Read the model definition and answer for the solid it produces. Units are mm, in the model's axes. Face numbers are marked on the shaded views. A direction names the side the tool comes from. Round coordinates to 2 decimals unless told otherwise and drop trailing zeros. Order: outer loops, then holes, each group sorted by start corner. A loop starts at its lowest first (then second) coordinate and runs counter-clockwise, first axis right, second up.
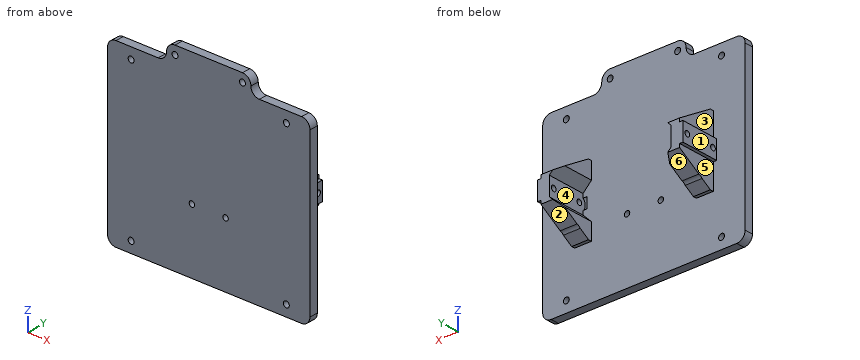
from build123d import *

# Parameters (mm, degrees)
EXTRUDE_1_DEPTH         = 5
FILLET_1_R              = 5
SKETCH_2_W              = 7
SKETCH_2_H              = 11
EXTRUDE_2_DEPTH         = 23
SKETCH_3_R              = 1.6
CUT_EXTRUDE_1_DEPTH     = 119.006186279
SKETCH_5_R              = 1.75
CUT_EXTRUDE_3_DEPTH     = 90.639556001
SKETCH_6_R              = 1.75
CUT_EXTRUDE_4_DEPTH     = 90.639556001
SKETCH2_R               = 4
CUT_EXTRUDE1_DEPTH      = 2.5
CUT_EXTRUDE2_START      = 2.5
SKETCH3_R               = 4
CUT_EXTRUDE2_DEPTH      = 2.5
CUT_EXTRUDE3_DEPTH      = 90.639556001
CUT_EXTRUDE3_DEPTH_BACK = 90.639556001
SKETCH4_R               = 1.6
EXTRUDE_4_DEPTH         = 5
EXTRUDE_4_DEPTH_BACK    = 5
EXTRUDE_5_DEPTH         = 5
EXTRUDE_5_DEPTH_BACK    = 5
CHAMFER_1_SIZE          = 5
SKETCH_12_R             = 1.6
EXTRUDE_6_DEPTH         = 5


with BuildPart() as part:
    # Sketch 1 → Extrude 1 (new body)
    with BuildSketch(Plane(origin=(0, 0, 0), x_dir=(1, 0, 0), z_dir=(0, 1, 0))):
        Polygon((-25, -52.5), (-60, -52.5), (-60, 52.5), (60, 52.5), (60, -52.5), (25, -52.5), (25, -62.5), (-25, -62.5), align=None)
    extrude(amount=EXTRUDE_1_DEPTH)

    # Fillet 1
    fillet_1_edges = [part.edges().sort_by_distance(p)[0] for p in [
        (60, 2.5, -52.5),
        (60, 2.5, 52.5),
        (-60, 2.5, -52.5),
        (-60, 2.5, 52.5),
        (-25, 2.5, 52.5),
        (25, 2.5, 52.5),
        (25, 2.5, 62.5),
        (-25, 2.5, 62.5),
    ]]
    fillet(fillet_1_edges, radius=FILLET_1_R - 0.0001)  # a hair under: the kernel refuses the full size

    # Sketch 5 → Cut-Extrude 3 (cut, through all)
    with BuildSketch(Plane(origin=(0, 5, 0), x_dir=(1, 0, 0), z_dir=(0, 1, 0))):
        with Locations(Location((-46, -46, 0), (0, 0, 270))):
            Circle(SKETCH_5_R)
        with Locations(Location((-46, 46, 0), (0, 0, 270))):
            Circle(SKETCH_5_R)
        with Locations(Location((46, 46, 0), (0, 0, 270))):
            Circle(SKETCH_5_R)
        with Locations(Location((46, -46, 0), (0, 0, 270))):
            Circle(SKETCH_5_R)
    extrude(amount=-CUT_EXTRUDE_3_DEPTH, mode=Mode.SUBTRACT)

    # Sketch 6 → Cut-Extrude 4 (cut, through all)
    with BuildSketch(Plane(origin=(0, 5, 0), x_dir=(1, 0, 0), z_dir=(0, 1, 0))):
        with Locations(Location((20, -57.5, 0), (0, 0, 270))):
            Circle(SKETCH_6_R)
        with Locations(Location((-20, -57.5, 0), (0, 0, 270))):
            Circle(SKETCH_6_R)
    extrude(amount=-CUT_EXTRUDE_4_DEPTH, mode=Mode.SUBTRACT)

    # Sketch2 → Cut-Extrude1 (cut)
    with BuildSketch(Plane.ZY.offset(-36.1)):
        with Locations((-0.7, 7.5)):
            Circle(SKETCH2_R)
    extrude(amount=CUT_EXTRUDE1_DEPTH, mode=Mode.SUBTRACT)

    # Sketch3 → Cut-Extrude2 (cut)
    with BuildSketch(Plane(origin=(-36.1, 0, 0), x_dir=(0, 0, -1), z_dir=(1, 0, 0)).offset(CUT_EXTRUDE2_START)):
        with Locations((0.7, 7.5)):
            Circle(SKETCH3_R)
    extrude(amount=-CUT_EXTRUDE2_DEPTH, mode=Mode.SUBTRACT)

    # Sketch4 → Cut-Extrude3 (cut, two sides: drawn at the far end of the back side and taken through both)
    with BuildSketch(Plane(origin=(0, 5, 0), x_dir=(1, 0, 0), z_dir=(0, 1, 0)).offset(-CUT_EXTRUDE3_DEPTH_BACK)):
        with Locations(Location((-10, 0, 0), (0, 0, 270))):
            Circle(SKETCH4_R)
        with Locations(Location((10, 0, 0), (0, 0, 270))):
            Circle(SKETCH4_R)
        with Locations(Location((-10, 14.7, 0), (0, 0, 270))):
            Circle(SKETCH4_R)
        with Locations(Location((10, 14.7, 0), (0, 0, 270))):
            Circle(SKETCH4_R)
    extrude(amount=CUT_EXTRUDE3_DEPTH + CUT_EXTRUDE3_DEPTH_BACK, mode=Mode.SUBTRACT)



with BuildPart() as body_2:
    # Sketch 2 → Extrude 2 (new body)
    with BuildSketch(Plane(origin=(0, 5, 0), x_dir=(1, 0, 0), z_dir=(0, 1, 0))):
        with Locations((-39.6, 0.7)):
            Rectangle(SKETCH_2_W, SKETCH_2_H)
    extrude(amount=EXTRUDE_2_DEPTH)

    # Sketch 3 → Cut-Extrude 1 (cut, through all)
    with BuildSketch(Plane(origin=(-36.1, 0, 0), x_dir=(0, 0, -1), z_dir=(1, 0, 0))):
        with Locations((0.7, 25)):
            Circle(SKETCH_3_R)
        with Locations((0.7, 7.5)):
            Circle(SKETCH_3_R)
    extrude(amount=-CUT_EXTRUDE_1_DEPTH, mode=Mode.SUBTRACT)


with BuildPart() as body_3:
    # Mirror 1: mirrored copy
    add(body_2.part.mirror(Plane(origin=(0, 0, 0), x_dir=(0, 0, 1), z_dir=(1, 0, 0))))


with BuildPart() as part_1:
    add(part.part)

    add(body_2.part)  # Extrude 4 merges body 2
    # Sketch 9 → Extrude 4 (add, two sides: drawn at the far end of the back side and taken through both)
    with BuildSketch(Plane(origin=(-36.1, 0, 0), x_dir=(0, 0, -1), z_dir=(1, 0, 0)).offset(-EXTRUDE_4_DEPTH_BACK)):
        Polygon((-19.8, 5), (-4.8, 5), (-4.8, 28), (-6.8, 28), (-19.8, 7), align=None)
        with BuildLine():
            Line((16.356233456, 14.824545956), (8.2, 28))
            Line((8.2, 28), (6.2, 28))
            Line((6.2, 28), (6.2, 5))
            Line((6.2, 5), (21.2, 5))
            Line((21.2, 5), (21.2, 7))
            Line((21.2, 7), (17.710979659, 12.636109782))
            ThreePointArc((17.710979659, 12.636109782), (16.87380684, 13.631404234), (16.356233456, 14.824545956))
        make_face()
    extrude(amount=EXTRUDE_4_DEPTH + EXTRUDE_4_DEPTH_BACK)


    add(body_3.part)  # Extrude 5 merges body 3
    # Sketch 10 → Extrude 5 (add, two sides: drawn at the far end of the back side and taken through both)
    with BuildSketch(Plane.ZY.offset(-36.1).offset(-EXTRUDE_5_DEPTH_BACK)):
        with BuildLine():
            Line((-21.2, 5), (-6.2, 5))
            Line((-6.2, 5), (-6.2, 28))
            Line((-6.2, 28), (-8.2, 28))
            Line((-8.2, 28), (-16.356233456, 14.824545956))
            ThreePointArc((-16.356233456, 14.824545956), (-16.87380684, 13.631404234), (-17.710979659, 12.636109782))
            Line((-17.710979659, 12.636109782), (-21.2, 7))
            Line((-21.2, 7), (-21.2, 5))
        make_face()
        Polygon((6.8, 28), (4.8, 28), (4.8, 5), (19.8, 5), (19.8, 7), align=None)
    extrude(amount=EXTRUDE_5_DEPTH + EXTRUDE_5_DEPTH_BACK)

    # Chamfer 1
    chamfer_1_edges = [part_1.edges().sort_by_distance(p)[0] for p in [
        (31.1, 16.5, 4.8),
        (31.1, 16.5, -6.2),
        (-31.1, 16.5, 4.8),
        (-31.1, 16.5, -6.2),
    ]]
    chamfer(chamfer_1_edges, length=CHAMFER_1_SIZE - 0.0001)  # a hair under: the kernel refuses the full size

    # Sketch 12 → Extrude 6 (add)
    with BuildSketch(Plane(origin=(0, 5, 0), x_dir=(1, 0, 0), z_dir=(0, 1, 0))):
        with Locations((-10, 0)):
            Circle(SKETCH_12_R)
        with Locations((10, 0)):
            Circle(SKETCH_12_R)
    extrude(amount=-EXTRUDE_6_DEPTH)


solid = part_1.part
Q1. For the marked faces 1, 2 and 3, determine the directions among +Z, -Z, +X, -X, +Y, -Y from which every point of the face is accessible in a straight line to the end or side of a thin tool.
Outcome:
face 1: +Z, -Z, -X, +Y
face 2: -Z, +X, -X, +Y
face 3: +Z, -X, +Y
Q2. A cutting plane is placed at A-A, the plane x = -10. Give the vertices of the cut face in (y, z), plus the area to 3 significant figures.
Outcome:
outline: (0, -52.5) - (5, -52.5) - (5, -16.3) - (0, -16.3) - close; (0, -13.1) - (5, -13.1) - (5, 62.5) - (0, 62.5) - close
area: 559 mm2
Q3. A cutting plane is placed at B-B, the plane x = -46. Give the vertices of the cut face in (y, z).
Outcome:
outline: (0, -52.5) - (5, -52.5) - (5, -47.75) - (0, -47.75) - close; (0, -44.25) - (5, -44.25) - (5, 44.25) - (0, 44.25) - close; (0, 47.75) - (5, 47.75) - (5, 52.5) - (0, 52.5) - close
Q4. A cutting plane is placed at D-D, the plane x = 53.5. Give the vertices of the cut face in (y, z).
Outcome:
outline: (0, -52.5) - (5, -52.5) - (5, 52.5) - (0, 52.5) - close
Q5. Straight lines are drawn through the part: probe 1 along X at (y, z) = (1.9, 57.5); probe 2 along X at (y, z) = (2.7, -46); probe 3 along X at (y, z) = (21.75, -3). For each, find the intervals that lie inside material, in ascending order.
Outcome:
probe 1: x = -25 to -21.75, -18.25 to 18.25, 21.75 to 25
probe 2: x = -60 to -47.75, -44.25 to 44.25, 47.75 to 60
probe 3: x = -43.1 to -36.1, 36.1 to 43.1
Q6. For a pull along Z with two mould halves and no side action, classify the marked faces 4, 5 and 6 as released by +Z, released by -Z, zero draft, split by the parting line, or undercut.
Outcome:
face 4: undercut
face 5: zero draft
face 6: released by -Z
Q7. Flat-ended cylindrical pins translate along their axes: pin 1 (0.6 mm diameter, centred on x = -42, y = 21, fed in from -Z); pin 2 (8 mm diameter, centred on y = 25, z = -7, fed in from -X); pin 3 (3 mm diameter, centred on y = 15.5, z = 16, fed in from -X); pin 4 (4 mm diameter, centred on x = -28, y = 8.5, fed in from -Z). Find the tip coordinate at first contact, or state that the pin passes through.
Outcome:
pin 1: stops at z = -6.2
pin 2: stops at x = -43.1
pin 3: stops at x = -41.1
pin 4: passes through
Q8. A cutting plane is placed at C-C, the plane y = 25. Give the number of separate pieces and of enclosed holes in the cut face, plus the area to 3 significant figures.
Outcome:
separate pieces: 4
enclosed holes: 0
area: 216 mm2
